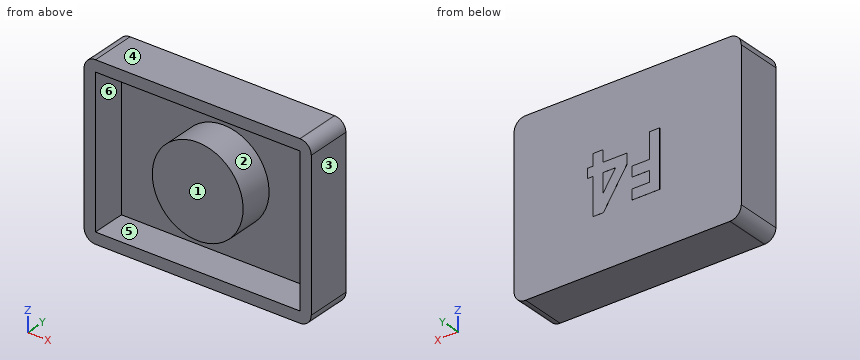
```python
from build123d import *

# Parameters (mm, degrees)
SKETCH1_W           = 12.7
SKETCH1_H           = 9.525
BOSS_EXTRUDE1_DEPTH = 2.54
FILLET1_R           = 0.635
SHELL1_START        = 0.635
SHELL1_OUTLINE_W    = 1.905
SHELL1_OUTLINE_H    = 8.255
SHELL1_DEPTH        = 11.43
SKETCH2_R           = 2.54
BOSS_EXTRUDE2_DEPTH = 1.905
BOSS_EXTRUDE3_DEPTH = 0.00254


# Read off the part's stored shape, not the designer's step: Shell1
with BuildPart() as part:
    # Sketch1 → Boss-Extrude1 (new body)
    with BuildSketch(Plane(origin=(0, 0, 0), x_dir=(1, 0, 0), z_dir=(0, 1, 0))):
        with Locations((6.35, 4.7625)):
            Rectangle(SKETCH1_W, SKETCH1_H)
    extrude(amount=BOSS_EXTRUDE1_DEPTH)

    # Fillet1
    fillet1_edges = [part.edges().sort_by_distance(p)[0] for p in [
        (0, 1.27, -9.525),
        (12.7, 1.27, -9.525),
        (12.7, 1.27, 0),
        (0, 1.27, 0),
    ]]
    fillet(fillet1_edges, radius=FILLET1_R)

    # Shell1 outline → Shell1 (cut)
    with BuildSketch(Plane.YZ.offset(SHELL1_START)):
        with Locations((0.9525, -4.7625)):
            Rectangle(SHELL1_OUTLINE_W, SHELL1_OUTLINE_H)
    extrude(amount=SHELL1_DEPTH, mode=Mode.SUBTRACT)

    # Sketch2 → Boss-Extrude2 (add)
    with BuildSketch(Plane(origin=(0, 1.905, 0), x_dir=(-1, 0, 0), z_dir=(0, -1, 0))):
        with Locations(Location((-6.35, 4.7625, 0), (0, 0, 270))):
            Circle(SKETCH2_R)
    extrude(amount=BOSS_EXTRUDE2_DEPTH)

    # Sketch3 → Boss-Extrude3 (add)
    # profile 1 of 2: a face of its own
    with BuildSketch(Plane(origin=(0, 2.54, 0), x_dir=(1, 0, 0), z_dir=(0, 1, 0))):
        Polygon((4.557346154, 6.477), (6.104141026, 6.477), (6.104141026, 5.907128205), (5.127217949, 5.907128205), (5.127217949, 5.296551282), (6.104141026, 5.296551282), (6.104141026, 4.726679487), (5.127217949, 4.726679487), (5.127217949, 3.302), (4.557346154, 3.302), align=None)
    # profile 2 of 2: a face of its own
    with BuildSketch(Plane(origin=(0, 2.54, 0), x_dir=(1, 0, 0), z_dir=(0, 1, 0))):
        Polygon((7.708177484, 6.558410256), (8.302217949, 6.558410256), (8.302217949, 4.482448718), (8.587153846, 4.482448718), (8.587153846, 3.953282051), (8.302217949, 3.953282051), (8.302217949, 3.302), (7.732346154, 3.302), (7.732346154, 3.953282051), (6.389076923, 3.953282051), (6.389076923, 4.53015004), align=None)
        Polygon((7.732346154, 4.482448718), (7.732346154, 5.563042668), (7.029546675, 4.482448718), align=None, mode=Mode.SUBTRACT)
    extrude(amount=BOSS_EXTRUDE3_DEPTH)


solid = part.part
```
For this review, take the finished solid that the model builds, in its own axes (mm). Face numbers are marked on the shaded views. A direction names the side the tool comes from. Round coordinates to 2 decimals unless told otherwise and drop trailing zeros. Order: outer loops, then holes, each group sorted by start corner. A loop starts at its lowest first (then second) coordinate and runs counter-clockwise, first axis right, second up.
Q1. Mouldability with a two-part tool opening along X and no side actions: class the marked faces 3, 4, 5 and 6 as pulls with the +X half, pulls with the -X half, needs draft (parallel to the pull), parting line crosses it, or undercut.
Findings below:
face 3: pulls with the +X half
face 4: needs draft
face 5: undercut
face 6: undercut
Q2. We need section A-A, the plane y = 1.15. State how many separate pieces and enclosed holes the cut face has, plus the area to 3 significant figures.
Findings below:
separate pieces: 2
enclosed holes: 1
area: 46.5 mm2
Q3. Wall thickness on line 1 (X direction, y = 0.6, z = -4.75) (3 decimals); line 2 (X direction, y = 0.7, z = -8.5) (3 decimals); line 3 (Z direction, x = 9.75, y = 1.2) (3 decimals): over which ranges is each line inside the solid? List them lowest first.
Findings below:
line 1: x = 0 to 0.635, 3.81 to 8.89, 12.065 to 12.7
line 2: x = 0 to 0.635, 12.065 to 12.7
line 3: z = -9.525 to -8.89, -0.635 to 0
Q4. We need section C-C, the plane x = 4. Give the boundary of the cut face in (y, z) (3 decimals), plus the area to 3 significant figures.
Findings below:
outline: (0, -9.525) - (2.54, -9.525) - (2.54, 0) - (0, 0) - (0, -0.635) - (1.905, -0.635) - (1.905, -3.799) - (0, -3.799) - (0, -5.726) - (1.905, -5.726) - (1.905, -8.89) - (0, -8.89) - close
area: 12.1 mm2
Q5. We need section B-B, the plane x = 10.75. Give the boundary of the cut face in (y, z) (3 decimals).
Findings below:
outline: (0, -9.525) - (2.54, -9.525) - (2.54, 0) - (0, 0) - (0, -0.635) - (1.905, -0.635) - (1.905, -8.89) - (0, -8.89) - close
Q6. Machinability: for the marked faces 1 and 2, which of the approach directions +Z, -Z, +X, -X, +Y, -Y give a long, thin tool a straight path to every point of the face, cutting with its end or side? Answer none if there is none.
Findings below:
face 1: +Z, -Z, +X, -X, -Y
face 2: -Y
Q7. Insertion check: P1, Ø4, axis at x = 6, z = -7, coming from the -Y side; P2, Ø2, axis at x = 2, z = -3, coming from the +Y side; P3, Ø1.5, axis at x = 11, z = -3, coming from the -Y side (3 decimals). Each pin has a flat end and moves straight along its axis. Give the tip position at first contact, or say it passes through.
Findings below:
P1: stops at y = 0
P2: stops at y = 2.54
P3: stops at y = 1.905
